The listing builds one solid part. Answer for the finished solid, in the listing's coordinates (mm). A direction names the side the tool comes from. Give positions to 0.01 mm unless a question says otherwise; leave off trailing zeros. Order: outer loops, then holes, each group sorted by start corner. A loop starts at its lowest first (then second) coordinate and runs counter-clockwise, first axis right, second up. Notation, with made-up numbers: (-18, -24.5) - (-14, -24.5) arc R24 cw to (-14, 6.5) - close; hole circle Ø3 at (-24, 24). An arc over 180 degrees is marked (long way). Write each question's results on one line, items separated by ' | '. Start each with the question number.
1. Find the intervals of material crossed by L1, parallel to X at y = -3.5, z = 2; L2, parallel to X at y = 9.75, z = 2.75; L3, parallel to Y at x = -23, z = 1, in increasing order.
2. Which of the six approach directions +Z, -Z, +X, -X, +Y, -Y give full straight-line access (tool end or side, diameter ignored) to faces 4 (the face through (-34, -6, 5)), 5 (the face through (-38, 0, 5)), 6 (the face through (-39.43, 5.4, 5.07)), 7 (the face through (-28, -1, 5)), 8 (the face through (34.5, 14, 5))?
3. Determine the mould class of faces 1 (the face through (-40, 0, 5)), 2 (the face through (30, 0, 5)), 3 (the face through (37, 6, 5)) for opening direction X: released by +X, released by -X, zero draft, split by the parting line, or undercut.
4. Section B-B (x = 23.5) is taken. Give the vertices of the cut face in (y, z).
5. Flat-ended cylindrical pins translate along their axes: pin 1 (0.8 mm diameter, centred on x = -37, z = 4, fed in from +Y); pin 2 (1.5 mm diameter, centred on y = 6, z = 1.5, fed in from +X). Find the tip coordinate at first contact, or state that the pin passes through.
6. Section D-D (z = 1.25) is taken. State how many separate pieces and enclosed holes the cut face has, and give its area (3 significant figures).
7. Section C-C (y = 7) is taken. Give the vertices of the cut face in (x, z), and give its area (3 significant figures).
8. Section A-A (y = -1.75) is taken. Give the vertices of the cut face in (x, z).
from build123d import *

# Parameters (mm, degrees)
F0_W     = 65
F0_H     = 15
F1_DEPTH = 10
F2_R     = 2


with BuildPart() as f1:
    # F0 (on Top) → F1 (new body)
    with BuildSketch(Plane.XY):
        Polygon((-40, -6), (-28, -6), (-28, 4), (28, 4), (28, -6), (40, -6), (40, 6), (34.5, 6), (34.5, 23), (-34.5, 23), (-34.5, 6), (-40, 6), align=None)
        Polygon((-38, 4), (-34.5, 4), (-30, 4), (-30, -4), (-38, -4), align=None, mode=Mode.SUBTRACT)
        Polygon((38, -4), (30, -4), (30, 4), (34.5, 4), (38, 4), align=None, mode=Mode.SUBTRACT)
        with Locations((0, 13.5)):
            Rectangle(F0_W, F0_H, mode=Mode.SUBTRACT)
    extrude(amount=F1_DEPTH)

    # F2
    f2_edges = [f1.edges().sort_by_distance(p)[0] for p in [
        (-34.5, 23, 5),
        (-40, 6, 5),
        (-40, -6, 5),
        (-28, -6, 5),
        (-28, 4, 5),
        (-34.5, 6, 5),
        (34.5, 23, 5),
        (34.5, 6, 5),
        (40, 6, 5),
        (40, -6, 5),
        (28, 4, 5),
        (28, -6, 5),
    ]]
    fillet(f2_edges, radius=F2_R)


solid = f1.part
Reported:
1) L1: -40 to -38, -30 to -28, 28 to 30, 38 to 40 | L2: -34.5 to -32.5, 32.5 to 34.5 | L3: 4 to 6, 21 to 23
2) face 4: +Z, -Z, +X, -X, -Y | face 5: +Z, -Z | face 6: +Z, -Z, -X, +Y | face 7: +Z, -Z, -Y | face 8: +Z, -Z, +X, +Y
3) face 1: released by -X | face 2: undercut | face 3: zero draft
4) outline: (4, 0) - (6, 0) - (6, 10) - (4, 10) - close; (21, 0) - (23, 0) - (23, 10) - (21, 10) - close
5) pin 1: y = 6 | pin 2: x = 39.56
6) separate pieces: 1 | enclosed holes: 3 | area: 467 mm²
7) outline: (-34.77, 0) - (-32.5, 0) - (-32.5, 10) - (-34.77, 10) - close; (32.5, 0) - (34.77, 0) - (34.77, 10) - (32.5, 10) - close | area: 45.4 mm²
8) outline: (-40, 0) - (-38, 0) - (-38, 10) - (-40, 10) - close; (-30, 0) - (-28, 0) - (-28, 10) - (-30, 10) - close; (28, 0) - (30, 0) - (30, 10) - (28, 10) - close; (38, 0) - (40, 0) - (40, 10) - (38, 10) - close
